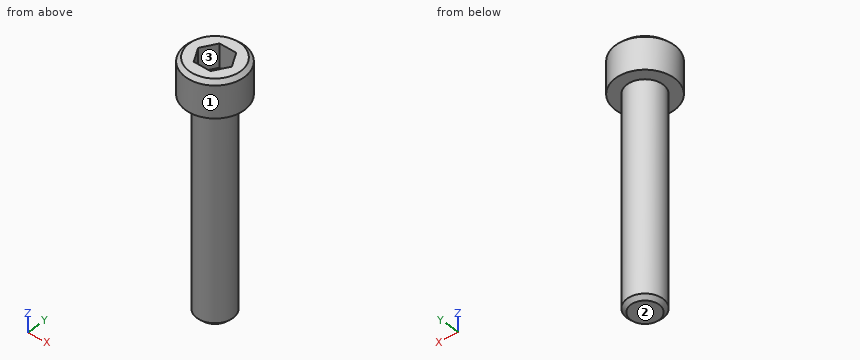
Autodesk Inventor part; units mm, degrees
ref_plane "YZ Plane" through (0, 0, 0) normal (1, 0, 0) x (0, 1, 0)
ref_plane "XZ Plane" through (0, 0, 0) normal (0, 1, 0) x (-1, 0, 0)
ref_plane "XY Plane" through (0, 0, 0) normal (0, 0, 1) x (1, 0, 0)
sketch "Sketch1" plane through (0, 0, 0) normal (0, 0, 1) x (1, 0, 0)
  circle A0 centre (0, 0) radius 3.9624
  dimension "d0" = 7.9248
extrude "Extrusion1" add sketch "Sketch1" along normal blind 4.826
sketch "Sketch2" plane through (0, 0, 0) normal (0, 0, -1) x (-1, 0, 0)
  circle A0 centre (0, 0) radius 3.9624
  circle A1 centre (0, 0) radius 2.413
  dimension "d3" = 4.826
extrude "Extrusion2" add sketch "Sketch2" along normal blind 28.575 contours A1
sketch "Sketch3" plane through (0, 0, 4.826) normal (0, 0, 1) x (1, 0, 0)
  circle A0 centre (0, 0) radius 3.9624
  line L0 (-1.1457, 1.9844) -> (1.1457, 1.9844)
  line L1 (1.1457, 1.9844) -> (2.2914, 0)
  line L2 (2.2914, 0) -> (1.1457, -1.9844)
  line L3 (1.1457, -1.9844) -> (-1.1457, -1.9844)
  line L4 (-1.1457, -1.9844) -> (-2.2914, 0)
  line L5 (-2.2914, 0) -> (-1.1457, 1.9844)
  dimension "d6" = 3.9688
extrude "Extrusion3" cut sketch "Sketch3" against normal blind 3.175 contours L0 L1 L2 L3 L4 L5
thread "Thread1"
chamfer "Chamfer1" distance 0.508 angle 45 1 edges at (2.413, 0, -28.575)
chamfer "Chamfer2" distance 0.508 angle 45 1 edges at (-3.9624, 0, 4.826)
properties part number "10-32 x1000" material "Steel"
The listing builds one solid part. Answer for the finished solid, in the listing's coordinates (mm). Face numbers are marked on the shaded views. Coordinates: 2 decimals unless noted, no trailing zeros. Order: outer loops, then holes, each group sorted by start corner. A loop starts at its lowest first (then second) coordinate and runs counter-clockwise, first axis right, second up. Notation, with made-up numbers: (-29.5, 79.5) -> (18.5, 79.5) arc R18 cw to (18.5, 113.5) -> close; hole circle Ø5 at (64, -22). An arc over 180 degrees is marked (long way). Answer in a Markdown table with one row per item. Add a question column.
Item 1: Find section B-B (z = -23). Write down the section's boundary in (x, y).
Item 2: Find the intervals of material crossed by L1, parallel to X at y = -0.75, z = -14.5; L2, parallel to Z at x = 2.75, y = -2, in increasing order. Write a range as from..to.
Item 3: Determine the mould class of the marked faces 1, 2 and 3 for opening direction Y: +Y half, -Y half, draft (parallel to the pull), parting line (faces both ways), or undercut.
Item 4: Find section A-A (x = 0). Write down the section's boundary in (y, z) (3 decimals), then the cut area to 3 significant figures.
Item 5: Each of these flat-tipped pins is pushed along its axis until it touches: P1, Ø1, axis at x = -3, y = -3, coming from the +Z side; P2, Ø2, axis at x = 0, z = -5.5, coming from the -Y side; P3, Ø1, axis at y = -2, z = -8.5, coming from the +X side. Where does it stop, or does it pass through?
Item 6: Find section C-C (z = 1). Write down the section's boundary in (x, y).
Result set:
| question | item | result |
|---|---|---|
| 1 | outline | circle Ø4.83 at (0, 0) |
| 2 | L1 | x = -2.29..2.29 |
| 2 | L2 | z = 0..4.83 |
| 3 | face 1 | parting line |
| 3 | face 2 | draft |
| 3 | face 3 | undercut |
| 4 | outline | (-3.962, 0) -> (-2.413, 0) -> (-2.413, -28.067) -> (-1.905, -28.575) -> (1.905, -28.575) -> (2.413, -28.067) -> (2.413, 0) -> (3.962, 0) -> (3.962, 4.318) -> (3.454, 4.826) -> (1.984, 4.826) -> (1.984, 1.651) -> (-1.984, 1.651) -> (-1.984, 4.826) -> (-3.454, 4.826) -> (-3.962, 4.318) -> close |
| 4 | area | 163 mm² |
| 5 | P1 | stops at z = 4.54 |
| 5 | P2 | stops at y = -2.41 |
| 5 | P3 | stops at x = 1.89 |
| 6 | outline | circle Ø7.92 at (0, 0) |
